```python
from build123d import *

# Parameters (mm, degrees)
F0_R     = 15.5321
F0_R_2   = 2.38125
F1_DEPTH = 42.3672
F3_DEPTH = 42.3672
F4_COUNT = 6
F4_ANGLE = 300


with BuildPart() as f1:
    # F0 (on Top) → F1 (new body)
    with BuildSketch(Plane.XY):
        Circle(F0_R)
        Circle(F0_R_2, mode=Mode.SUBTRACT)
    extrude(amount=F1_DEPTH)

    # F2 (on face) → F3 (cut, through all)
    with BuildSketch(Plane.XY.offset(42.3672)):
        with BuildLine():
            ThreePointArc((-1.5474074833, 1.8099396794), (-1.190625, 2.0622229928), (-0.79375, 2.2450640303))
            Line((-0.79375, 2.2450640303), (-0.79375, 13.9219908812))
            ThreePointArc((-0.79375, 13.9219908812), (-3.6091280563, 13.4694492773), (-6.2735877764, 12.4536727744))
            Line((-6.2735877764, 12.4536727744), (-2.38125, 5.7119459855))
            ThreePointArc((-2.38125, 5.7119459855), (-3.0942155106, 5.3593384739), (-3.7560653285, 4.9181959855))
            Line((-3.7560653285, 4.9181959855), (-7.6484031049, 11.6599227744))
            ThreePointArc((-7.6484031049, 11.6599227744), (-9.8603212209, 9.8603212209), (-11.6599227744, 7.6484031049))
            Line((-11.6599227744, 7.6484031049), (-1.5474074833, 1.8099396794))
        make_face()
    f3 = extrude(amount=-F3_DEPTH, mode=Mode.SUBTRACT)

    # F4: F3 ×6 about axis
    f4_axis = Axis((0, 0, 0), (0, 0, 1))
    for i in range(1, F4_COUNT):
        add(f3.rotate(f4_axis, i * F4_ANGLE / (F4_COUNT - 1)), mode=Mode.SUBTRACT)


solid = f1.part
```
Work out the finished part from the listing and answer in its coordinate system (mm). Coordinates: 2 decimals unless noted, no trailing zeros. Write each loop counter-clockwise with the first axis right and the second up, starting at its lowest first coordinate (ties: lowest second). Pieces come first, ordered by that corner, then holes.
Q1. Find the intervals of material crossed by line 1 (Y direction, x = -12, z = 22); line 2 (Y direction, x = 9, z = 10.5), in increasing order.
Q2. A cutting plane is placed at B-B, the plane x = -5. Give the vertices of the cut face in (y, z), then the cut area to 3 significant figures.
Q3. A cutting plane is placed at A-A, the plane x = 0. Give the vertices of the cut face in (y, z).
Q4. Each of these flat-tipped pins is pushed along its axis until it touches: pin 1 Ø2.5 at (x, z) = (-11, 15.5) entering from +Y; pin 2 Ø2.5 at (x, z) = (9, 15) entering from -Y; pin 3 Ø13 at (y, z) = (10.5, 12.5) entering from -X. Where does it stop, or does it pass through?
Q5. A cutting plane is placed at C-C, the plane y = -9. Give the vertices of the cut face in (x, z), then the cut area to 3 significant figures.
Findings below:
1. line 1: y = -9.86 to -6.01, -0.79 to 0.79, 6.01 to 9.86
1. line 2: y = -12.66 to -10.65, -6.11 to -4.28, -0.79 to 0.79, 4.28 to 6.11, 10.65 to 12.66
2. outline: (-14.71, 0) - (-13.02, 0) - (-13.02, 42.37) - (-14.71, 42.37) - close; (-10.25, 0) - (-7.07, 0) - (-7.07, 42.37) - (-10.25, 42.37) - close; (-3.8, 0) - (-1.97, 0) - (-1.97, 42.37) - (-3.8, 42.37) - close; (1.97, 0) - (3.8, 0) - (3.8, 42.37) - (1.97, 42.37) - close; (7.07, 0) - (10.25, 0) - (10.25, 42.37) - (7.07, 42.37) - close; (13.02, 0) - (14.71, 0) - (14.71, 42.37) - (13.02, 42.37) - close
2. area: 567 mm2
3. outline: (-15.53, 0) - (-2.38, 0) - (-2.38, 42.37) - (-15.53, 42.37) - close; (2.38, 0) - (15.53, 0) - (15.53, 42.37) - (2.38, 42.37) - close
4. pin 1: stops at y = 12.09
4. pin 2: stops at y = -13.46
4. pin 3: stops at x = -15.01
5. outline: (-12.66, 0) - (-10.65, 0) - (-10.65, 42.37) - (-12.66, 42.37) - close; (-6.11, 0) - (-4.28, 0) - (-4.28, 42.37) - (-6.11, 42.37) - close; (-0.79, 0) - (0.79, 0) - (0.79, 42.37) - (-0.79, 42.37) - close; (4.28, 0) - (6.11, 0) - (6.11, 42.37) - (4.28, 42.37) - close; (10.65, 0) - (12.66, 0) - (12.66, 42.37) - (10.65, 42.37) - close
5. area: 393 mm2
